For this review, take the finished solid that the model builds, in its own axes (mm). A direction names the side the tool comes from. Give positions to 0.01 mm unless a question says otherwise; leave off trailing zeros. Loops run counter-clockwise (first coordinate to the right, second up) from the corner with the lowest first, then second, coordinate; pieces in that order, holes last. Notation, with made-up numbers: (-8, 36) -> (43, 36) arc R17 ccw to (43, 66) -> close; hole circle Ø5 at (72, 66). An arc over 180 degrees is marked (long way). Answer as CSV lines item,"result". Start each with the question number.
Item 1: Add section B-B on x = -16.5. State the section outline as (y, z) points.
Item 2: Add section A-A on z = 16. State the section outline as (x, y) points.
Item 3: Add section C-C on y = -25. State the section outline as (x, z) points.
Item 4: Clearance check with flat-ended pins moving along their axes: P1, Ø11.5, axis at x = 5.5, y = -27, coming from the +Z side; P2, Ø6, axis at x = -25, z = -12.5, coming from the -Y side; P3, Ø11.5, axis at x = 7.5, y = 26.5, coming from the -Z side; P4, Ø10.5, axis at y = -22, z = 7.5, coming from the +X side. State where each tip first meets the part, or that it passes through.
Item 5: Add section D-D on x = 28. State the section outline as (y, z) points.
Item 6: For L1, parallel to Z at x = 12, y = -29; L2, parallel to X at y = 20.5, z = -7.5; L3, parallel to Y at x = 27.5, z = -16, list the stretches that pass through material, from the lowest coordinate up. Write a range as from..to.
Item 7: Machinability: for faces 1 (the face through (-22.5, 23, 0)), 2 (the face through (22.5, 23, 0)), 3 (the face through (-22.5, -23, 0)), 4 (the face through (0, 25, -20)), 5 (the face through (22.5, -23, 0)), which of the approach directions +Z, -Z, +X, -X, +Y, -Y give a long, thin tool a straight path to every point of the face, cutting with its end or side? Answer none if there is none.
```python
from build123d import *

# Parameters (mm, degrees)
SKETCH001_W  = 45
SKETCH001_H  = 65
PAD001_DEPTH = 20
FILLET_R     = 5
SKETCH_W     = 66
SKETCH_H     = 55
PAD_DEPTH    = 18


with BuildPart() as coil:
    # Sketch001 → Pad001 (new body, symmetric)
    with BuildSketch(Plane.XY):
        Rectangle(SKETCH001_W, SKETCH001_H)
    extrude(amount=PAD001_DEPTH, both=True)

    # Fillet
    fillet_edges = [coil.edges().sort_by_distance(p)[0] for p in [
        (-22.5, -32.5, 0),
        (22.5, -32.5, 0),
        (22.5, 32.5, 0),
        (-22.5, 32.5, 0),
    ]]
    fillet(fillet_edges, radius=FILLET_R)


with BuildPart() as fusion_of_core_and_coil:
    # Sketch → Pad (new body, symmetric)
    with BuildSketch(Plane.XZ):
        Rectangle(SKETCH_W, SKETCH_H)
    extrude(amount=PAD_DEPTH, both=True)

    # Fusion: union Coil
    add(coil.part)


solid = fusion_of_core_and_coil.part
```
Computed values:
1,outline,"(-32.5, -20) -> (-18, -20) -> (-18, -27.5) -> (18, -27.5) -> (18, -20) -> (32.5, -20) -> (32.5, 20) -> (18, 20) -> (18, 27.5) -> (-18, 27.5) -> (-18, 20) -> (-32.5, 20) -> close"
2,outline,"(-33, -18) -> (-22.5, -18) -> (-22.5, -27.5) arc R5 ccw to (-17.5, -32.5) -> (17.5, -32.5) arc R5 ccw to (22.5, -27.5) -> (22.5, -18) -> (33, -18) -> (33, 18) -> (22.5, 18) -> (22.5, 27.5) arc R5 ccw to (17.5, 32.5) -> (-17.5, 32.5) arc R5 ccw to (-22.5, 27.5) -> (-22.5, 18) -> (-33, 18) -> close"
3,outline,"(-22.5, -20) -> (22.5, -20) -> (22.5, 20) -> (-22.5, 20) -> close"
4,P1,"z = 20"
4,P2,"y = -29.68"
4,P3,"z = -20"
4,P4,"x = 33"
5,outline,"(-18, -27.5) -> (18, -27.5) -> (18, 27.5) -> (-18, 27.5) -> close"
6,L1,"-20..20"
6,L2,"-22.5..22.5"
6,L3,"-18..18"
7,face 1,"+Z, -Z, -X, +Y"
7,face 2,"+Z, -Z, +X, +Y"
7,face 3,"+Z, -Z, -X, -Y"
7,face 4,"-Z, +X, -X, +Y"
7,face 5,"+Z, -Z, +X, -Y"
